Autodesk Fusion 360 part; units mm, degrees
sketch "Skizze1" plane through (0, 0, 0) normal (0, 0, 1) x (1, 0, 0)
  point P0 (-5.2, 16.4)
sketch "Skizze2" plane through (0, 0, 0) normal (0, 0, 1) x (1, 0, 0)
  circle A0 centre (0, 0) radius 6
extrude "Extrusion2" add sketch "Skizze2" along normal blind 110
sketch "Skizze3" plane through (0, 0, 0) normal (0, 0, 1) x (1, 0, 0)
  line L0 (-1.5, -2) -> (-1.5, 2)
  line L1 (1.5, -2) -> (1.5, 2)
  arc A0 (-1.5, -2) -> (1.5, -2) centre (0, 0) ccw
  arc A1 (1.5, 2) -> (-1.5, 2) centre (0, 0) ccw
  dimension "d15" = 5
extrude "Extrusion3" cut sketch "Skizze3" along normal blind 20
pattern_linear "R-Anordnung1" count 2 spacing 98 along (0, 0, 1) of "Extrusion3"
ref_plane "Arbeitsebene1" through (-6, 0, 108.0306) normal (-1, 0, 0) x (0, 1, 0)
sketch "Skizze5" plane through (-6, 0, 0) normal (-1, 0, 0) x (0, -1, 0)
  line L0 (0, 110) -> (-6.178, 103.822)
  line L1 (-6.178, 103.822) -> (-6.178, 110)
  line L2 (-6.178, 110) -> (0, 110)
extrude "Extrusion4" cut sketch "Skizze5" against normal blind 100
Build history of the part. All positions in model axes, mm. A direction names the side the tool comes from. Round coordinates to 2 decimals unless told otherwise and drop trailing zeros. Write each loop counter-clockwise with the first axis right and the second up, starting at its lowest first coordinate (ties: lowest second). Pieces come first, ordered by that corner, then holes. Notation, with made-up numbers: (45.5, 11) -> (84.5, 11) arc R28 ccw to (84.5, 46) -> close; hole circle Ø10 at (31.5, 8.5). An arc over 180 degrees is marked (long way). Put each result on its own line as item: value.
Item 1: Wall check: probe 1 along X at (y, z) = (1.5, 14.5); probe 2 along Z at (x, y) = (-1, 2); probe 3 along X at (y, z) = (2, 102). Give the ranges that are in metal, low to high. Write a range as from..to.
Here are the results:
probe 1: x = -5.81..-1.5, 1.5..5.81
probe 2: z = 20..98
probe 3: x = -5.66..-1.5, 1.5..5.66
Item 2: Slice it at A-A, the plane x = 0. Give the cut face in (y, z), plus the area to 3 significant figures.
Here are the results:
outline: (-6, 0) -> (-2.5, 0) -> (-2.5, 20) -> (2.5, 20) -> (2.5, 0) -> (6, 0) -> (6, 104) -> (2.5, 107.5) -> (2.5, 98) -> (-2.5, 98) -> (-2.5, 110) -> (-6, 110) -> close
area: 1,150 mm^2
Item 3: Slice it at D-D, the plane x = -4. Give the cut face in (y, z), plus the area to 3 significant figures.
Here are the results:
outline: (-4.47, 0) -> (4.47, 0) -> (4.47, 105.53) -> (0, 110) -> (-4.47, 110) -> close
area: 974 mm^2
Item 4: Slice it at B-B, the plane z = 57. Give the cut face in (x, y), plus the area to 3 significant figures.
Here are the results:
outline: circle Ø12 at (0, 0)
area: 113 mm^2
Item 5: Two-plate mould, pull along Y, no slides. Class faces 4 (the face through (0, -3, 110)), 5 (the face through (0, 3, 107)), 6 (the face through (1.5, 0, 104)): pulls with the +Y half, pulls with the -Y half, needs draft (parallel to the pull), parting line crosses it, or undercut.
Here are the results:
face 4: needs draft
face 5: pulls with the +Y half
face 6: undercut
Item 6: Slice it at C-C, the plane x = 5. Give the cut face in (y, z).
Here are the results:
outline: (-3.32, 0) -> (3.32, 0) -> (3.32, 106.68) -> (0, 110) -> (-3.32, 110) -> close
Item 7: Tool access for faces 1 (the face through (-6, 0, 54)), 2 (the face through (1.5, 0, 10)), 3 (the face through (0, -2.5, 103.9)): list every direction of +Z, -Z, +X, -X, +Y, -Y with a clear straight run to the whole face (end or side of a thin tool).
Here are the results:
face 1: +Z, -Z
face 2: -Z
face 3: +Z
Item 8: Flat gauge pins, fed straight in: P1, Ø5, axis at y = 4, z = 59, coming from the -X side; P2, Ø1.5, axis at x = 0.5, y = 0, coming from the +Z side; P3, Ø1.2, axis at y = 0.5, z = 103, coming from the -X side; P4, Ø1, axis at x = 1, z = 25.5, coming from the +Y side. Where does each tip first touch, or does it go through?
Here are the results:
P1: stops at x = -5.81
P2: stops at z = 98
P3: stops at x = -6
P4: stops at y = 5.98
